```python
from build123d import *

# Parameters (mm, degrees)
SKETCH1_W           = 152.4
SKETCH1_H           = 152.4
SKETCH1_R           = 6.35
BOSS_EXTRUDE1_DEPTH = 6.35
SKETCH2_W           = 50.4
SKETCH2_H           = 101.6
BOSS_EXTRUDE2_DEPTH = 76.2
SKETCH3_R           = 6.35
BOSS_EXTRUDE3_DEPTH = 6.35
FILLET2_R           = 5
FILLET6_R           = 5


with BuildPart() as part:
    # Sketch1 → Boss-Extrude1 (new body)
    with BuildSketch(Plane.XY):
        with Locations((76.2, 76.2)):
            Rectangle(SKETCH1_W, SKETCH1_H)
        with Locations((25.4, 127)):
            Circle(SKETCH1_R, mode=Mode.SUBTRACT)
        with Locations((127, 127)):
            Circle(SKETCH1_R, mode=Mode.SUBTRACT)
        with Locations((127, 25.4)):
            Circle(SKETCH1_R, mode=Mode.SUBTRACT)
        with Locations((25.4, 25.4)):
            Circle(SKETCH1_R, mode=Mode.SUBTRACT)
    extrude(amount=BOSS_EXTRUDE1_DEPTH)

    # Sketch2 → Boss-Extrude2 (add)
    with BuildSketch(Plane.XY.offset(6.35)):
        with Locations((76.4, 76.2)):
            Rectangle(SKETCH2_W, SKETCH2_H)
    extrude(amount=BOSS_EXTRUDE2_DEPTH)

    # Sketch3 → Boss-Extrude3 (add)
    with BuildSketch(Plane.XY.offset(82.55)):
        Polygon((101.6, 152.4), (152.4, 152.4), (152.4, 0), (101.6, 0), (101.6, 25.4), (50.8, 25.4), (50.8, 0), (0, 0), (0, 152.4), (50.8, 152.4), (50.8, 127), (101.6, 127), align=None)
        with Locations((25.4, 127)):
            Circle(SKETCH3_R, mode=Mode.SUBTRACT)
        with Locations((127, 127)):
            Circle(SKETCH3_R, mode=Mode.SUBTRACT)
        with Locations((127, 25.4)):
            Circle(SKETCH3_R, mode=Mode.SUBTRACT)
        with Locations((25.4, 25.4)):
            Circle(SKETCH3_R, mode=Mode.SUBTRACT)
    extrude(amount=BOSS_EXTRUDE3_DEPTH)

    # Fillet2
    fillet2_edges = [part.edges().sort_by_distance(p)[0] for p in [
        (76.4, 25.4, 6.35),
        (51.2, 76.2, 6.35),
        (76.4, 127, 6.35),
        (101.6, 76.2, 6.35),
    ]]
    fillet(fillet2_edges, radius=FILLET2_R)

    # Fillet6
    fillet6_edges = [part.edges().sort_by_distance(p)[0] for p in [
        (76.2, 25.4, 88.9),
        (76.2, 127, 88.9),
    ]]
    fillet(fillet6_edges, radius=FILLET6_R)


solid = part.part
```
Work out the finished part from the listing and answer in its coordinate system (mm). A direction names the side the tool comes from. Round coordinates to 2 decimals unless told otherwise and drop trailing zeros. Loops run counter-clockwise (first coordinate to the right, second up) from the corner with the lowest first, then second, coordinate; pieces in that order, holes last.
(1) The part is cut by section B-B, the plane x = 140.5. Give the vertices of the cut face in (y, z).
Computed values:
outline: (0, 0) - (152.4, 0) - (152.4, 6.35) - (0, 6.35) - close; (0, 82.55) - (152.4, 82.55) - (152.4, 88.9) - (0, 88.9) - close
(2) The part is cut by section D-D, the plane y = 130. Give the number of separate pieces and of enclosed holes in the cut face, and give its area (3 significant figures).
Computed values:
separate pieces: 7
enclosed holes: 0
area: 1,350 mm2
(3) The part is cut by section A-A, the plane x = 25.4. Give the vertices of the cut face in (y, z).
Computed values:
outline: (0, 0) - (19.05, 0) - (19.05, 6.35) - (0, 6.35) - close; (0, 82.55) - (19.05, 82.55) - (19.05, 88.9) - (0, 88.9) - close; (31.75, 0) - (120.65, 0) - (120.65, 6.35) - (31.75, 6.35) - close; (31.75, 82.55) - (120.65, 82.55) - (120.65, 88.9) - (31.75, 88.9) - close; (133.35, 0) - (152.4, 0) - (152.4, 6.35) - (133.35, 6.35) - close; (133.35, 82.55) - (152.4, 82.55) - (152.4, 88.9) - (133.35, 88.9) - close
(4) The mould has two halves that part along X. Classify faces 1 (the flat face through (127, 0, 86)), 2 (the flat face through (152.4, 77, 86)), 3 (the cylindrical face through (20.36, 21.54, 3.13)), 4 (the flat face through (51.2, 75, 46)): pulls with the +X half, pulls with the -X half, needs draft (parallel to the pull), parting line crosses it, or undercut.
Computed values:
face 1: needs draft
face 2: pulls with the +X half
face 3: undercut
face 4: pulls with the -X half
(5) For faces 5 (the flat face through (77, 77, 88.9)), 6 (the cylindrical face through (103.03, 76.98, 7.85)), 7 (the flat face through (101.6, 12, 86)), 8 (the cylindrical face through (76.56, 125.57, 87.4)), determine the directions among +Z, -Z, +X, -X, +Y, -Y from which every point of the face is accessible in a straight line to the end or side of a thin tool.
Computed values:
face 5: +Z, +X, -X, +Y, -Y
face 6: +X, +Y, -Y
face 7: +Z, -Y
face 8: +Z, +Y
(6) The part is cut by section C-C, the plane y = 109. Give the vertices of the cut face in (x, z).
Computed values:
outline: (0, 0) - (152.4, 0) - (152.4, 6.35) - (106.6, 6.35) arc R5 cw to (101.6, 11.35) - (101.6, 82.55) - (152.4, 82.55) - (152.4, 88.9) - (0, 88.9) - (0, 82.55) - (51.2, 82.55) - (51.2, 11.35) arc R5 cw to (46.2, 6.35) - (0, 6.35) - close
(7) Each of these flat-tipped pins is pushed along its axis until it touches: P1, Ø4, axis at y = 51, z = 53, coming from the -X side; P2, Ø5, axis at x = 69.5, z = 12, coming from the +Y side; P3, Ø11.5, axis at x = 127, y = 25.4, coming from the -Z side; P4, Ø5, axis at x = 84, z = 31.5, coming from the -Y side. Where does it stop, or does it pass through?
Computed values:
P1: stops at x = 51.2
P2: stops at y = 127.35
P3: passes through
P4: stops at y = 25.4
(8) Find the intervals of material crossed by L1, parallel to X at y = 25, z = 86; L2, parallel to Z at x = 38.5, y = 94.5; L3, parallel to Y at x = 25.4, z = 84.75, in increasing order.
Computed values:
L1: x = 0 to 19.06, 31.74 to 50.8, 101.6 to 120.66, 133.34 to 152.4
L2: z = 0 to 6.35, 82.55 to 88.9
L3: y = 0 to 19.05, 31.75 to 120.65, 133.35 to 152.4
